Read the model definition and answer for the solid it produces. Units are mm, in the model's axes. A direction names the side the tool comes from. Coordinates: 2 decimals unless noted, no trailing zeros. Loops run counter-clockwise (first coordinate to the right, second up) from the corner with the lowest first, then second, coordinate; pieces in that order, holes last. Notation, with made-up numbers: (65, 53) - (117, 53) arc R35 ccw to (117, 90) - close; hole circle Ø7 at (-13.5, -9.75). An arc over 180 degrees is marked (long way). One line per question, with ' | ' between items. Start each with the question number.
```python
from build123d import *
from build123d.topology import SkipClean

# Parameters (mm, degrees)
SKETCH_1_R      = 3.5
EXTRUDE_1_DEPTH = 10
EXTRUDE_START   = 10
EXTRUDE_2_DEPTH = 10


with BuildPart() as part:
    # Эскиз1 → Бобышка-Вытянуть1 (new body)
    with BuildSketch(Plane(origin=(0, 0, 0), x_dir=(1, 0, 0), z_dir=(0, 1, 0))):
        with BuildLine():
            Line((5.196152423, 0), (17.897858345, 0))
            ThreePointArc((17.897858345, 0), (20.495934556, 1.5), (20.495934556, 4.5))
            Line((20.495934556, 4.5), (14.145081595, 15.5))
            ThreePointArc((14.145081595, 15.5), (11.547005384, 17), (8.948929172, 15.5))
            Line((8.948929172, 15.5), (2.598076211, 4.5))
            ThreePointArc((2.598076211, 4.5), (2.598076211, 1.5), (5.196152423, 0))
        make_face()
        with Locations(Location((15.299782134, 4.5, 0), (0, 0, 270))):
            Circle(SKETCH_1_R, mode=Mode.SUBTRACT)
        with Locations(Location((11.547005384, 11, 0), (0, 0, 270))):
            Circle(SKETCH_1_R, mode=Mode.SUBTRACT)
        with Locations(Location((7.794228634, 4.5, 0), (0, 0, 270))):
            Circle(SKETCH_1_R, mode=Mode.SUBTRACT)
    extrude(amount=EXTRUDE_1_DEPTH)

    # Эскиз4 → Бобышка-Вытянуть2 (add)
    with SkipClean():  # the faces are left unmerged after this step: merging them gives an invalid solid
        with BuildSketch(Plane(origin=(0, 0, 0), x_dir=(-1, 0, 0), z_dir=(0, -1, 0)).offset(EXTRUDE_START)):
            with BuildLine():
                Line((-5.196152423, 0), (-17.803847577, 0))
                ThreePointArc((-17.803847577, 0), (-20.401923789, 1.5), (-20.401923789, 4.5))
                Line((-20.401923789, 4.5), (-14.098076211, 15.418584287))
                ThreePointArc((-14.098076211, 15.418584287), (-11.5, 16.918584287), (-8.901923789, 15.418584287))
                Line((-8.901923789, 15.418584287), (-2.598076211, 4.5))
                ThreePointArc((-2.598076211, 4.5), (-2.598076211, 1.5), (-5.196152423, 0))
            make_face()
            with BuildLine():
                Line((-7.794228634, 1), (-15.299782134, 1))
                ThreePointArc((-15.299782134, 1), (-18.330871047, 2.75), (-18.330871047, 6.25))
                Line((-18.330871047, 6.25), (-14.578094297, 12.75))
                ThreePointArc((-14.578094297, 12.75), (-11.547005384, 14.5), (-8.515916471, 12.75))
                Line((-8.515916471, 12.75), (-4.763139721, 6.25))
                ThreePointArc((-4.763139721, 6.25), (-4.763139721, 2.75), (-7.794228634, 1))
            make_face(mode=Mode.SUBTRACT)
        extrude(amount=-EXTRUDE_2_DEPTH)


solid = part.part
```
1) Which of the six approach directions +Z, -Z, +X, -X, +Y, -Y give full straight-line access (tool end or side, diameter ignored) to faces 1 (the cylindrical face through (11.6, 4.9, -17)), 2 (the flat face through (11, -5, -1)), 3 (the flat face through (17.294, -5.07, -9.883)), 4 (the cylindrical face through (20.4, -5.1, -1.5))?
2) Find the intervals of material crossed by line 1 along X through (y, z) = (4.25, -4.5); line 2 along Z through (x, y) = (14, 4.25); line 3 along Z through (x, y) = (11, 2.25), in increasing order. Write a range as from..to.
3) The part is cut by section B-B on x = 16.25. Write down the section's boundary in (y, z).
4) The mould has two halves that part along X. Classify faces 5 (the flat face through (6.67, -5.07, -9.55)), 6 (the cylindrical face through (11.54, -5.07, -16.92)), 7 (the flat face through (12, 10, -7)): released by +X, released by -X, zero draft, split by the parting line, or undercut.
5) The part is cut by section C-C on z = -9.5. Write down the section's boundary in (x, y).
6) The part is cut by section A-A on y = -2.25. Write down the section's boundary in (x, z).
7) Given pin 1 Ø4 at (y, z) = (6.5, -14) entering from -X; pin 2 Ø1 at (x, z) = (4, -7) entering from -Y; pin 3 Ø4 at (x, z) = (15.3, -4.5) entering from -Y; pin 4 Ø2 at (y, z) = (-2.5, -6) entering from -X, each flat-ended and moving along its own axis, determine where each tip first touches the part or whether it passes through.
8) The part is cut by section D-D on x = 12.75. Write down the section's boundary in (y, z), and give its area (3 significant figures).
Answer below:
1) face 1: -Z, +Y, -Y | face 2: -Y | face 3: -Z, +X, -Y | face 4: +X, -Y
2) line 1: 2.6..4.29, 11.29..11.8, 18.8..20.5 | line 2: -15.73..-13.5, -8.5..-7.75, -1.25..0 | line 3: -16.95..-14.46, -7.54..-5.9, -3.1..0
3) outline: (-10, -11.69) - (0, -11.69) - (0, -11.85) - (10, -11.85) - (10, -7.87) - (0, -7.87) - (0, -9.85) - (-10, -9.85) - close; (-10, -1.13) - (10, -1.13) - (10, 0) - (-10, 0) - close
4) face 5: undercut | face 6: split by the parting line | face 7: zero draft
5) outline: (5.48, -10) - (6.64, -10) - (6.64, 0) - (8.38, 0) - (8.38, 10) - (5.48, 10) - close; (14.71, 0) - (16.45, 0) - (16.45, -10) - (17.52, -10) - (17.52, 0) - (17.61, 0) - (17.61, 10) - (14.71, 10) - close
6) outline: (2.6, -4.5) - (8.9, -15.42) arc R3 ccw to (14.1, -15.42) - (20.4, -4.5) arc R3 ccw to (17.8, 0) - (5.2, 0) arc R3 ccw to start; hole (4.76, -6.25) - (8.52, -12.75) arc R3.5 ccw to (14.58, -12.75) - (18.33, -6.25) arc R3.5 ccw to (15.3, -1) - (7.79, -1) arc R3.5 ccw to start
7) pin 1: x = 6.93 | pin 2: y = -10 | pin 3: through | pin 4: x = 2.89
8) outline: (-10, -16.65) - (0, -16.65) - (0, -16.75) - (10, -16.75) - (10, -14.29) - (-10, -14.29) - close; (-10, -1) - (0, -1) - (0, -2.1) - (10, -2.1) - (10, 0) - (-10, 0) - close; (0, -7.71) - (10, -7.71) - (10, -6.9) - (0, -6.9) - close | area: 87.4 mm2
